Autodesk Inventor part; units mm, degrees
ref_plane "YZ Plane" through (0, 0, 0) normal (1, 0, 0) x (0, 1, 0)
ref_plane "XZ Plane" through (0, 0, 0) normal (0, 1, 0) x (-1, 0, 0)
ref_plane "XY Plane" through (0, 0, 0) normal (0, 0, 1) x (1, 0, 0)
sketch "Sketch1" plane through (0, 0, 0) normal (0, 1, 0) x (-1, 0, 0)
  line L0 (0, -37.5) -> (4.5, -37.5) construction
  line L1 (0, 0) -> (2, 0) construction
  line L2 (4.5, -37.5) -> (6.5, -37.5) construction
  line L3 (0, -75) -> (2, -75) construction
  arc A0 (2.4733, -73) -> (3.9166, -9) centre (-152, -37.5) ccw
  line L4 (1.9166, -9) -> (3.9166, -9)
  line L5 (0, -73) -> (2.4733, -73)
  line L6 (0, -15) -> (2.8949, -15) construction
  line L7 (0, -67) -> (1.7305, -67) construction
  line L8 (0, -69) -> (1.3383, -69) construction
  line L9 (1.3383, -69) -> (1.3383, -67)
  line L10 (1.3383, -67) -> (1.7305, -67)
  arc A1 (2.2393, -10.8253) -> (1.9166, -9) centre (-154, -37.5) ccw
  arc A2 (0.4733, -73) -> (0.9193, -71) centre (-154, -37.5) ccw
  arc A3 (1.7305, -67) -> (2.8949, -15) centre (-154, -37.5) ccw
  line L11 (-6.1617, -13) -> (-6.1617, -11)
  line L12 (-6.1617, -11) -> (-6.1617, -10.8253)
  line L13 (-6.1617, -10.8253) -> (2.2393, -10.8253)
  line L14 (1.3383, -67) -> (1.3383, -5.3327) construction
  line L15 (2.8949, -15) -> (1.3383, -15) construction
  line L16 (2.8949, -15) -> (1.3383, -15)
  line L17 (1.3383, -15) -> (1.3383, -13)
  line L18 (1.3383, -13) -> (-6.1617, -13)
  line L19 (1.3383, -69) -> (-6.1617, -69)
  line L20 (-6.1617, -69) -> (-6.1617, -71)
  line L21 (-6.1617, -71) -> (0.9193, -71)
  arc A4 (2.8949, -15) -> (2.2393, -10.8253) centre (-154, -37.5) ccw
  line L22 (1.3383, -13) -> (2.595, -13)
  arc A5 (0.9193, -71) -> (1.7305, -67) centre (-154, -37.5) ccw
  line L23 (1.3383, -15) -> (1.3383, -67)
  line L24 (-6.1617, -13) -> (-6.1617, -69)
  line L25 (2.8949, -15) -> (4.8949, -15)
  line L26 (1.7305, -67) -> (3.7305, -67)
  point P0 (0, -7)
  point P1 (2, 0)
  point P2 (0, -9)
  point P3 (0, -41)
  point P4 (0, -13)
  dimension "d14" = 75
  dimension "d15" = 4.5
  dimension "d16" = 68
  dimension "d17" = 2
  dimension "d18" = 2
  dimension "d19" = 2
  dimension "d20" = 2
  dimension "d21" = 2
  dimension "d22" = 32
  dimension "d23" = 26
  dimension "d24" = 26
  dimension "d26" = 28
  dimension "d27" = 28
  dimension "d29" = 2
  dimension "d30" = 7.5
  dimension "d31" = 7.5
  dimension "d32" = 2
extrude "Extrusion1" add sketch "Sketch1" along normal blind 138 contours L5 A2 A5 L26 A0 | L26 A3 L25 A0 | L25 A4 A1 L4 A0
extrude "Extrusion2" add sketch "Sketch1" along normal blind 133 contours A5 L9 L10 | L10 L23 L16 A3 | L21 L20 L19 A5 | L16 L17 L22 A4 | L9 L19 L24 L18 L17 L23 | L22 L18 L11 L12 L13 A4
extrude "Extrusion3" cut sketch "Sketch1" along normal blind 131 contours L10 L23 L16 A3 | L9 L19 L24 L18 L17 L23
extrude "Extrusion4" cut sketch "Sketch1" along normal blind 129 contours L26 A3 L25 A0
extrude "Extrusion5" add sketch "Sketch1" along normal blind 131 contours L10 L23 L16 A3
extrude "Extrusion6" cut sketch "Sketch1" along normal blind 129 contours L10 L23 L16 A3
extrude "Extrusion7" add sketch "Sketch1" along normal blind 51 contours L26 A3 L25 A0
extrude "Extrusion8" add sketch "Sketch1" along normal blind 51 contours L10 L23 L16 A3
extrude "Extrusion9" cut sketch "Sketch1" along normal blind 43 contours A5 L9 L10 | L10 L23 L16 A3 | L16 L17 L22 A4 | L9 L19 L24 L18 L17 L23
properties part number "facet"
Can you work these out from the model? Positions are in its coordinate system, mm. A direction names the side the tool comes from. Give positions to 0.01 mm unless a question says otherwise; leave off trailing zeros. Loops run counter-clockwise (first coordinate to the right, second up) from the corner with the lowest first, then second, coordinate; pieces in that order, holes last. Notation, with made-up numbers: (50, 7.25) -> (64, 7.25) arc R11 cw to (64, 16.25) -> close; hole circle Ø4 at (55, 53.5). An arc over 180 degrees is marked (long way). Return JSON: item names as keys, results as strings.
Q1. For pin 1 Ø6 at (x, z) = (4, -35.5) entering from -Y; pin 2 Ø3.5 at (x, y) = (4, 50.5) entering from -Z; pin 3 Ø1.6 at (x, z) = (-3.5, -31.5) entering from -Y, each with a flat end and sliding along its axis, tell me the tip position at first contact or that it passes through.
Checks:
{"pin 1": "stops at y = 131", "pin 2": "stops at z = -71", "pin 3": "stops at y = 43"}
Q2. I want a section at B-B, the plane y = 67. List the corners of the cut face in (x, z) for me, then the cut area to 3 significant figures.
Checks:
{"outline": "(-4.89, -15) -> (-1.34, -15) -> (-1.34, -13) -> (6.16, -13) -> (6.16, -10.83) -> (-2.24, -10.83) arc R156.47 cw to (-1.92, -9) -> (-3.92, -9) arc R158.5 ccw to start; (-3.73, -67) arc R158.5 ccw to (-2.47, -73) -> (-0.47, -73) arc R157.68 cw to (-0.92, -71) -> (6.16, -71) -> (6.16, -69) -> (-1.34, -69) -> (-1.34, -67) -> close", "area": "60.5 mm2"}
Q3. I want a section at A-A, the plane z = -22. List the corners of the cut face in (x, y) for me, then the cut area to 3 significant figures.
Checks:
{"outline": "(-5.74, 0) -> (-3.74, 0) -> (-3.74, 43) -> (-1.34, 43) -> (-1.34, 51) -> (-5.74, 51) -> close; (-5.74, 129) -> (-1.34, 129) -> (-1.34, 131) -> (6.16, 131) -> (6.16, 133) -> (-3.74, 133) -> (-3.74, 138) -> (-5.74, 138) -> close", "area": "164 mm2"}
Q4. I need wall thicknesses on probe 1 along Y at (x, z) = (-2.5, -18); probe 2 along Z at (x, y) = (4.5, 130); probe 3 along Y at (x, z) = (-6, -30). Which ranges of each line are inside material? Lowest first, please.
Checks:
{"probe 1": "y = 43 to 51, 129 to 133", "probe 2": "z = -71 to -69, -13 to -10.83", "probe 3": "y = 0 to 51, 129 to 138"}
Q5. We'd pull the mould along Z, two halves only. Please class faces 1 (the face through (2, 65, -69)), 2 (the face through (-6.47, 37.37, -40.62)), 3 (the face through (6.162, 66, -12)): released by +Z, released by -Z, zero draft, split by the parting line, or undercut.
Checks:
{"face 1": "undercut", "face 2": "split by the parting line", "face 3": "zero draft"}
Q6. I want a section at D-D, the plane y = 19.5. List the corners of the cut face in (x, z) for me (1 decimal), then the cut area to 3 significant figures.
Checks:
{"outline": "(-3.9, -9) arc R158.5 ccw to (-2.5, -73) -> (-0.5, -73) arc R157.7 cw to (-0.9, -71) -> (6.2, -71) -> (6.2, -69) -> (-1.3, -69) arc R158.5 cw to (-1.7, -67) arc R158.5 cw to (-2.9, -15) arc R158.5 cw to (-2.6, -13) -> (6.2, -13) -> (6.2, -10.8) -> (-2.2, -10.8) arc R156.5 cw to (-1.9, -9) -> close", "area": "161 mm2"}
Q7. I want a section at C-C, the plane z = -52. List the corners of the cut face in (x, y) for me.
Checks:
{"outline": "(-5.84, 0) -> (-3.84, 0) -> (-3.84, 43) -> (-1.34, 43) -> (-1.34, 51) -> (-5.84, 51) -> close; (-5.84, 129) -> (-1.34, 129) -> (-1.34, 131) -> (6.16, 131) -> (6.16, 133) -> (-3.84, 133) -> (-3.84, 138) -> (-5.84, 138) -> close"}
Q8. On a 3-axis mill with a long thin cutter (end or side, diameter ignored), from which of +Z, -Z, +X, -X, +Y, -Y can I reach the whole of each face in a straight line? I mean faces 4 (the face through (-2.576, 135.465, -12.881)), 5 (the face through (-3, 89, -15)), 6 (the face through (-1.343, 135.465, -68.975)), 7 (the face through (-3, 43, -41)). Say none if no direction works.
Checks:
{"face 4": "+X, +Y", "face 5": "+X, -X", "face 6": "+Z, +X, +Y", "face 7": "+X, -Y"}
